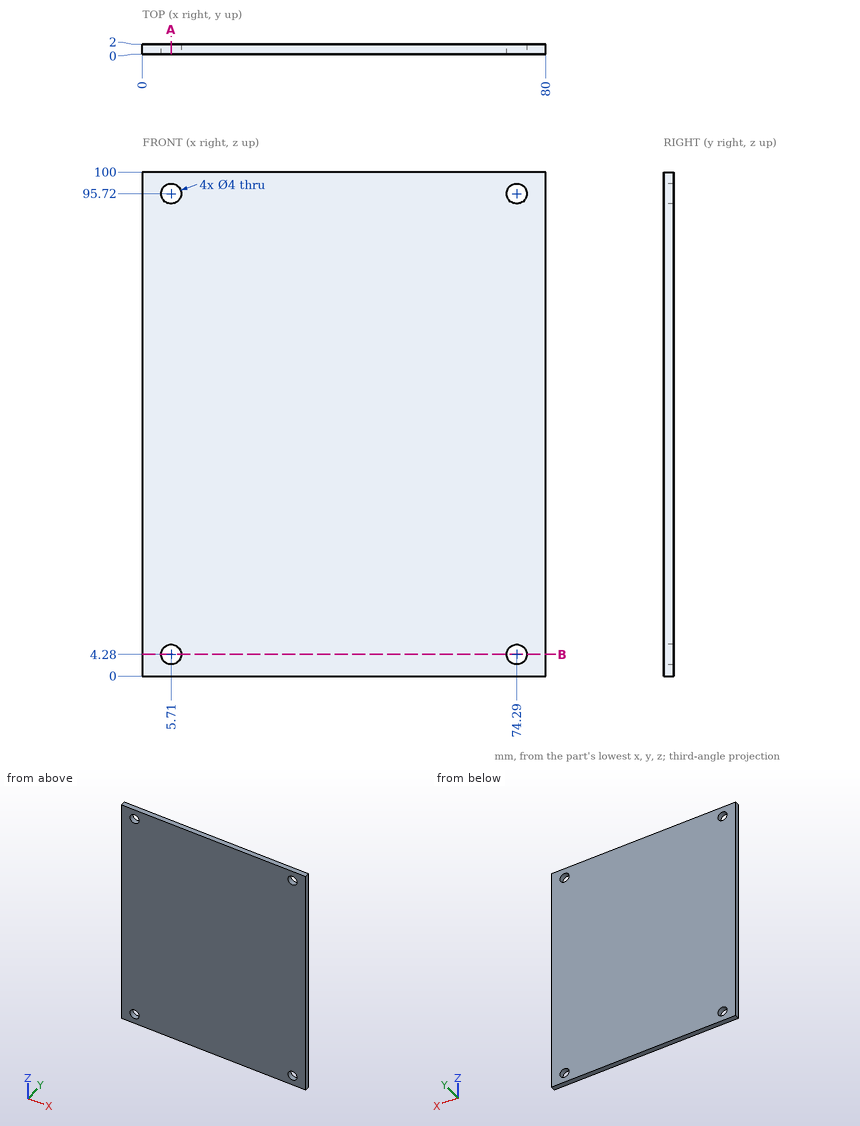
The drawing under review shows one solid part. Ordinate dimensions are in mm from its lowest x, y, z. Coordinates: 2 decimals unless noted, no trailing zeros. Loops run counter-clockwise (first coordinate to the right, second up) from the corner with the lowest first, then second, coordinate; pieces in that order, holes last. Notation, with made-up numbers: M 47.25,-35 L 70.25,-35 A17 cw 70.25,-22 Z; hole C -23.5,27.5 d7. An arc over 180 degrees is marked long. Use one line per item in the form item = value.
(1) Consider section A-A (x = 5.71). Write out the cut boundary in (y, z), and give its area (3 significant figures).
Return value:
outline = M 0,0 L 2,0 L 2,2.28 L 0,2.28 Z; M 0,6.28 L 2,6.28 L 2,93.72 L 0,93.72 Z; M 0,97.72 L 2,97.72 L 2,100 L 0,100 Z
area = 184 mm2
(2) Clearance check with a flat-ended pin moving along its axis: P1, Ø3.5, axis at x = 5.71, z = 4.28, coming from the +Y side. State where the tip first meets the part, or that it passes through.
Return value:
P1 = through
(3) Consider section B-B (z = 4.28). Write out the cut boundary in (x, y).
Return value:
outline = M 0,0 L 3.71,0 L 3.71,2 L 0,2 Z; M 7.71,0 L 72.29,0 L 72.29,2 L 7.71,2 Z; M 76.29,0 L 80,0 L 80,2 L 76.29,2 Z
(4) For line 1 along Z through (x, y) = (74.29, 1.05), list the stretches that pass through material, from the lowest coordinate up. Write a range as from..to.
Return value:
line_1 = 0..2.28, 6.28..93.72, 97.72..100
